```python
from build123d import *

# Parameters (mm, degrees)
ESQUISSE1_R             = 2
BOSS_EXTRU_1_DEPTH      = 6
ENL_V_MAT_EXTRU_1_REACH = 142.485
ESQUISSE2_W             = 40
ESQUISSE2_H             = 10


with BuildPart() as part:
    # Esquisse1 → Boss.-Extru.1 (new body)
    with BuildSketch(Plane(origin=(0, 0, 0), x_dir=(1, 0, 0), z_dir=(0, 1, 0))):
        Polygon((0, 0), (140, 0), (140, 10), (-140, 10), (-140, 0), align=None)
        with Locations(Location((-135, 5, 0), (0, 0, 270))):
            Circle(ESQUISSE1_R, mode=Mode.SUBTRACT)
        with Locations(Location((-125, 5, 0), (0, 0, 270))):
            Circle(ESQUISSE1_R, mode=Mode.SUBTRACT)
        with Locations(Location((-115, 5, 0), (0, 0, 270))):
            Circle(ESQUISSE1_R, mode=Mode.SUBTRACT)
        with Locations(Location((-105, 5, 0), (0, 0, 270))):
            Circle(ESQUISSE1_R, mode=Mode.SUBTRACT)
        with Locations(Location((-95, 5, 0), (0, 0, 270))):
            Circle(ESQUISSE1_R, mode=Mode.SUBTRACT)
        with Locations(Location((-85, 5, 0), (0, 0, 270))):
            Circle(ESQUISSE1_R, mode=Mode.SUBTRACT)
        with Locations(Location((-75, 5, 0), (0, 0, 270))):
            Circle(ESQUISSE1_R, mode=Mode.SUBTRACT)
        with Locations(Location((-65, 5, 0), (0, 0, 270))):
            Circle(ESQUISSE1_R, mode=Mode.SUBTRACT)
        with Locations(Location((-55, 5, 0), (0, 0, 270))):
            Circle(ESQUISSE1_R, mode=Mode.SUBTRACT)
        with Locations(Location((-45, 5, 0), (0, 0, 270))):
            Circle(ESQUISSE1_R, mode=Mode.SUBTRACT)
        with Locations(Location((-35, 5, 0), (0, 0, 270))):
            Circle(ESQUISSE1_R, mode=Mode.SUBTRACT)
        with Locations(Location((-25, 5, 0), (0, 0, 270))):
            Circle(ESQUISSE1_R, mode=Mode.SUBTRACT)
        with Locations(Location((-15, 5, 0), (0, 0, 270))):
            Circle(ESQUISSE1_R, mode=Mode.SUBTRACT)
        with Locations(Location((-5, 5, 0), (0, 0, 270))):
            Circle(ESQUISSE1_R, mode=Mode.SUBTRACT)
        with Locations(Location((5, 5, 0), (0, 0, 270))):
            Circle(ESQUISSE1_R, mode=Mode.SUBTRACT)
        with Locations(Location((15, 5, 0), (0, 0, 270))):
            Circle(ESQUISSE1_R, mode=Mode.SUBTRACT)
        with Locations(Location((25, 5, 0), (0, 0, 270))):
            Circle(ESQUISSE1_R, mode=Mode.SUBTRACT)
        with Locations(Location((35, 5, 0), (0, 0, 270))):
            Circle(ESQUISSE1_R, mode=Mode.SUBTRACT)
        with Locations(Location((45, 5, 0), (0, 0, 270))):
            Circle(ESQUISSE1_R, mode=Mode.SUBTRACT)
        with Locations(Location((55, 5, 0), (0, 0, 270))):
            Circle(ESQUISSE1_R, mode=Mode.SUBTRACT)
        with Locations(Location((65, 5, 0), (0, 0, 270))):
            Circle(ESQUISSE1_R, mode=Mode.SUBTRACT)
        with Locations(Location((75, 5, 0), (0, 0, 270))):
            Circle(ESQUISSE1_R, mode=Mode.SUBTRACT)
        with Locations(Location((85, 5, 0), (0, 0, 270))):
            Circle(ESQUISSE1_R, mode=Mode.SUBTRACT)
        with Locations(Location((95, 5, 0), (0, 0, 270))):
            Circle(ESQUISSE1_R, mode=Mode.SUBTRACT)
        with Locations(Location((105, 5, 0), (0, 0, 270))):
            Circle(ESQUISSE1_R, mode=Mode.SUBTRACT)
        with Locations(Location((115, 5, 0), (0, 0, 270))):
            Circle(ESQUISSE1_R, mode=Mode.SUBTRACT)
        with Locations(Location((125, 5, 0), (0, 0, 270))):
            Circle(ESQUISSE1_R, mode=Mode.SUBTRACT)
        with Locations(Location((135, 5, 0), (0, 0, 270))):
            Circle(ESQUISSE1_R, mode=Mode.SUBTRACT)
    extrude(amount=BOSS_EXTRU_1_DEPTH)

    # Esquisse2 → Enlèv. mat.-Extru.1 (cut, up to next)
    with BuildSketch(Plane(origin=(0, 6, 0), x_dir=(1, 0, 0), z_dir=(0, 1, 0)), mode=Mode.PRIVATE) as enl_v_mat_extru_1_sk1:
        with Locations((120, 5)):
            Rectangle(ESQUISSE2_W, ESQUISSE2_H)
    enl_v_mat_extru_1_tool1 = extrude(enl_v_mat_extru_1_sk1.sketch, amount=-ENL_V_MAT_EXTRU_1_REACH, mode=Mode.PRIVATE) & part.part
    add(enl_v_mat_extru_1_tool1.solids().sort_by_distance((120, 6, -5))[0], mode=Mode.SUBTRACT)


solid = part.part
```
CAD build for the part. Positions are in the model's coordinates, mm. Give positions to 0.01 mm unless a question says otherwise; leave off trailing zeros. Write each loop counter-clockwise with the first axis right and the second up, starting at its lowest first coordinate (ties: lowest second). Pieces come first, ordered by that corner, then holes. Notation, with made-up numbers: M -22,38.5 L 16,38.5 A7 cw 16,45.5 Z; hole C -31,12.5 d4. An arc over 180 degrees is marked long. Return JSON: item names as keys, results as strings. Group by question number.
(1) Band-saw the part on B-B (y = 1.25). State how many separate pieces and enclosed holes the cut face has, and give its area (3 significant figures).
(2) Drill centre lines: L1, parallel to Z at x = -135, y = 3.8; L2, parallel to Z at x = -46, y = 4.6. Where is each one in solid material? Low to high. Write a range as [from, to].
(3) Band-saw the part on A-A (x = -35). Give the cut face in (y, z), and give its area (3 significant figures).
(4) Flat gauge pin, fed straight in: pin 1 Ø1 at (x, z) = (1.5, -7.5) entering from -Y. Where does the tip first touch, or does it go through?
(5) Mould opens along Z. For faces 1 (the face through (-22, 3, 0)), 2 (the face through (-83, 3, -5)), 3 (the face through (-22, 0, -5)) say: pulls with the +Z half, pulls with the -Z half, needs draft (parallel to the pull), parting line crosses it, or undercut.
Entries:
{
 "1": {"separate pieces": "1", "enclosed holes": "24", "area": "2,100 mm^2"},
 "2": {"L1": "z = [-10, -7], [-3, 0]", "L2": "z = [-10, -6.73], [-3.27, 0]"},
 "3": {"outline": "M 0,-10 L 6,-10 L 6,-7 L 0,-7 Z; M 0,-3 L 6,-3 L 6,0 L 0,0 Z", "area": "36.0 mm^2"},
 "4": {"pin 1": "stops at y = 0"},
 "5": {"face 1": "pulls with the +Z half", "face 2": "undercut", "face 3": "needs draft"}
}
